For this review, take the finished solid that the model builds, in its own axes (mm). A direction names the side the tool comes from. Coordinates: 2 decimals unless noted, no trailing zeros. Write each loop counter-clockwise with the first axis right and the second up, starting at its lowest first coordinate (ties: lowest second). Pieces come first, ordered by that corner, then holes. Notation, with made-up numbers: M 36.5,66.5 L 72.5,66.5 A15 ccw 72.5,74.5 Z; hole C -29,-1.75 d3. An arc over 180 degrees is marked long. One line per question, with ' | ' between items.
from build123d import *

# Parameters (mm, degrees)
SKETCH1_W           = 24
SKETCH1_H           = 18
SKETCH1_W_2         = 1.5
SKETCH1_H_2         = 12
SKETCH1_W_3         = 1.75
SKETCH1_W_4         = 7
SKETCH1_H_3         = 3
BOSS_EXTRUDE1_DEPTH = 5.5
FILLET1_R           = 3
FILLET2_R           = 3
FILLET4_R           = 1.5
FILLET5_R           = 1.5


with BuildPart() as part:
    # Sketch1 → Boss-Extrude1 (new body)
    with BuildSketch(Plane(origin=(0, 0, 0), x_dir=(1, 0, 0), z_dir=(0, 1, 0))):
        with Locations((-12, 9)):
            Rectangle(SKETCH1_W, SKETCH1_H)
        with Locations((-13.25, 9)):
            Rectangle(SKETCH1_W_2, SKETCH1_H_2, mode=Mode.SUBTRACT)
        with Locations((-20.625, 9)):
            Rectangle(SKETCH1_W_3, SKETCH1_H_2, mode=Mode.SUBTRACT)
        with Locations((-5.5, 14)):
            Rectangle(SKETCH1_W_4, SKETCH1_H_3, mode=Mode.SUBTRACT)
        with Locations((-5.5, 4)):
            Rectangle(SKETCH1_W_4, SKETCH1_H_3, mode=Mode.SUBTRACT)
    extrude(amount=BOSS_EXTRUDE1_DEPTH)

    # Fillet1
    fillet1_edges = [part.edges().sort_by_distance(p)[0] for p in [
        (0, 2.75, 0),
    ]]
    fillet(fillet1_edges, radius=FILLET1_R)

    # Fillet2
    fillet2_edges = [part.edges().sort_by_distance(p)[0] for p in [
        (-24, 2.75, 0),
        (-24, 2.75, -18),
        (0, 2.75, -18),
    ]]
    fillet(fillet2_edges, radius=FILLET2_R)

    # Fillet4
    fillet4_edges = [part.edges().sort_by_distance(p)[0] for p in [
        (-9, 2.75, -15.5),
        (-9, 2.75, -5.5),
        (-9, 2.75, -12.5),
        (-9, 2.75, -2.5),
        (-2, 2.75, -2.5),
    ]]
    fillet(fillet4_edges, radius=FILLET4_R - 0.0001)  # a hair under: the kernel refuses the full size

    # Fillet5
    fillet5_edges = [part.edges().sort_by_distance(p)[0] for p in [
        (-2, 2.75, -12.5),
        (-2, 2.75, -5.5),
        (-2, 2.75, -15.5),
    ]]
    fillet(fillet5_edges, radius=FILLET5_R - 0.0001)  # a hair under: the kernel refuses the full size


solid = part.part
1) We need section C-C on z = -12. State the section outline as (x, y) points, then the cut area to 3 significant figures.
Responses:
outline: M -24,0 L -21.5,0 L -21.5,5.5 L -24,5.5 Z; M -19.75,0 L -14,0 L -14,5.5 L -19.75,5.5 Z; M -12.5,0 L 0,0 L 0,5.5 L -12.5,5.5 Z | area: 114 mm^2
2) Machinability: for faces 1 (the flat face through (-13, 3, -15)), 2 (the cylindrical face through (-0.86, 2.79, -17.1)), which of the approach directions +Z, -Z, +X, -X, +Y, -Y give a long, thin tool a straight path to every point of the face, cutting with its end or side? Answer none if there is none.
Responses:
face 1: +Y, -Y | face 2: -Z, +X, +Y, -Y
3) We need section D-D on x = -20.5. State the section outline as (y, z) points, then the cut area to 3 significant figures.
Responses:
outline: M 0,-18 L 5.5,-18 L 5.5,-15 L 0,-15 Z; M 0,-3 L 5.5,-3 L 5.5,0 L 0,0 Z | area: 33.0 mm^2
4) We need section B-B on y = 4.45. State how many separate pieces and enclosed holes the cut face has, then the cut area to 3 significant figures.
Responses:
separate pieces: 1 | enclosed holes: 4 | area: 347 mm^2
5) To check wall thickness, follow line 1 along X through (y, z) = (4.7, -8.5); line 2 along Z through (x, y) = (-4.5, 1.8); line 3 along X through (y, z) = (1.55, -4.5). State the ranges of each line that lie inside material, in increasing order. Write a range as [from, to].
Responses:
line 1: [-24, -21.5], [-19.75, -14], [-12.5, 0] | line 2: [-18, -15.5], [-12.5, -5.5], [-2.5, 0] | line 3: [-24, -21.5], [-19.75, -14], [-12.5, -8.91], [-2.09, 0]
6) The part is to be moulded in two halves that separate along X. For faces 3 (the flat face through (-12, 5.5, -9)), 4 (the cylindrical face through (-23.14, 2.79, -17.1)), 5 (the cylindrical face through (-8.55, 2.79, -5.07)), say which applies: +X half, -X half, draft (parallel to the pull), parting line (faces both ways), or undercut.
Responses:
face 3: draft | face 4: -X half | face 5: undercut
7) We need section A-A on x = -4.75. State the section outline as (y, z) points.
Responses:
outline: M 0,-18 L 5.5,-18 L 5.5,-15.5 L 0,-15.5 Z; M 0,-12.5 L 5.5,-12.5 L 5.5,-5.5 L 0,-5.5 Z; M 0,-2.5 L 5.5,-2.5 L 5.5,0 L 0,0 Z
